from build123d import *
from build123d.topology import SkipClean

# Parameters (mm, degrees)
SKETCH_1_R          = 7.75
EXTRUDE_1_DEPTH     = 1.5
SKETCH_2_R          = 6.5
EXTRUDE_2_DEPTH     = 4
SKETCH_4_W          = 19
SKETCH_4_H          = 19
CUT_EXTRUDE_1_DEPTH = 1
SKETCH_5_R          = 0.4
EXTRUDE_3_DEPTH     = 5.1
FILLET_1_R          = 0.4
FILLET_2_R          = 1


with BuildPart() as part:
    # 草图1 → 凸台-拉伸1 (new body)
    with BuildSketch(Plane.XY):
        Circle(SKETCH_1_R)
    extrude(amount=EXTRUDE_1_DEPTH)

    # 草图2 → 凸台-拉伸2 (add)
    with BuildSketch(Plane.XY.offset(1.5)):
        Circle(SKETCH_2_R)
    extrude(amount=EXTRUDE_2_DEPTH)

    # 草图4 → 切除-拉伸1 (cut)
    with BuildSketch(Plane.XY.offset(5.5)):
        Rectangle(SKETCH_4_W, SKETCH_4_H)
        Polygon((-2.5, 7.5), (-2.5, 2.5), (-7.5, 2.5), (-7.5, -2.5), (-2.5, -2.5), (-2.5, -7.5), (2.5, -7.5), (2.5, -2.5), (7.5, -2.5), (7.5, 2.5), (2.5, 2.5), (2.5, 7.5), align=None, mode=Mode.SUBTRACT)
    extrude(amount=-CUT_EXTRUDE_1_DEPTH, mode=Mode.SUBTRACT)

    # 草图3 → 切除-旋转2 (revolve, cut)
    with SkipClean():  # the faces are left unmerged after this step: merging them gives an invalid solid
        with BuildSketch(Plane(origin=(0, 0, 0), x_dir=(1, 0, 0), z_dir=(0, 1, 0)), mode=Mode.PRIVATE) as cut_revolve_2_sk:
            with BuildLine():
                Line((-6.5, -5.5), (0, -5.5))
                Line((0, -5.5), (0, -4.735087663))
                ThreePointArc((0, -4.735087663), (-3.272426122, -4.926973248), (-6.5, -5.5))
            make_face()
            with BuildLine():
                Line((0, -4.735087663), (0, -5.5))
                Line((0, -5.5), (6.5, -5.5))
                ThreePointArc((6.5, -5.5), (3.272426122, -4.926973248), (0, -4.735087663))
            make_face()
        revolve(cut_revolve_2_sk.sketch.rotate(Axis((0, 0, 1000), (0, 0, -1)), 337.380135052), axis=Axis((0, 0, 1000), (0, 0, -1)), mode=Mode.SUBTRACT)
    add(part.part.scale(1), mode=Mode.REPLACE)  # the faces are merged on a copy

    # 草图5 → 凸台-拉伸3 (add)
    with BuildSketch(Plane(origin=(0, 0, 0), x_dir=(-1, 0, 0), z_dir=(0, 0, -1))):
        Circle(SKETCH_5_R)
    extrude(amount=-EXTRUDE_3_DEPTH)

    # 圆角1
    # the kernel refuses this fillet: 0.4 mm, written as the material it takes off along each edge
    with BuildSketch(Plane(origin=(0, 0, 5.1), x_dir=(-1, 0, 0), z_dir=(0, -1, 0))) as fillet_1_piece_1:
        with BuildLine():
            CenterArc((0.001803842, 0.4), FILLET_1_R, 270, 84.556601085)
            Line((0.001803842, 0), (0.001803842, -0.008))
            Line((0.001803842, -0.008), (0.4, -0.008))
            Line((0.4, -0.008), (0.408, 0))
            ThreePointArc((0.408, 0), (0.408, 0.181027524), (0.407963923, 0.36129615))
            Line((0.407963923, 0.36129615), (0.4, 0.362055049))
        make_face()
    revolve(axis=Axis((0, 0, 5.1), (0, 0, -1)), mode=Mode.SUBTRACT)

    # 圆角2
    fillet_2_edges = [part.edges().sort_by_distance(p)[0] for p in [
        (2.5, 2.5, 4.729599419),
        (2.5, -2.5, 4.729599419),
        (-2.5, -2.5, 4.729599419),
        (-2.5, 2.5, 4.729599419),
    ]]
    fillet(fillet_2_edges, radius=FILLET_2_R)


solid = part.part
For this review, take the finished solid that the model builds, in its own axes (mm). A direction names the side the tool comes from. Give positions to 0.01 mm unless a question says otherwise; leave off trailing zeros. Order: outer loops, then holes, each group sorted by start corner. A loop starts at its lowest first (then second) coordinate and runs counter-clockwise, first axis right, second up. Notation, with made-up numbers: M 48.5,17 L 102.5,17 A23 ccw 102.5,46 Z; hole C 43.25,-15 d11. An arc over 180 degrees is marked long. Answer in a Markdown table with one row per item. Add a question column.
(1) Mouldability with a two-part tool opening along Z and no side actions: class faces 6 (the face through (0, 0, 0)), 7 (the face through (4, 4, 4.5)), 8 (the face through (-5, -2.5, 5)) as +Z half, -Z half, draft (parallel to the pull), parting line (faces both ways), or undercut.
(2) Consider section C-C on z = 3.4. State the section outline as (x, y) points.
(3) Consider section D-D on y = -5. State the section outline as (x, z) points.
(4) For faces 1 (the face through (5, -2.5, 5)), 2 (the face through (6.2, 1.95, 3.47)), 3 (the face through (-2.801, 2.785, 4.78)), 4 (the face through (-2.785, -2.801, 4.78)), 5 (the face through (5, 2.5, 5)), list the 3-axis set-ups (+Z, -Z, +X, -X, +Y, -Y) from which the entire face can be reached by the end or side of a thin tool; tool diameter is ignored.
(5) Consider section A-A on y = 4.25. State the section outline as (x, z) points, and give its area (3 significant figures).
(6) Consider section B-B on x = 1.75. State the section outline as (y, z) points.
(7) For pin 1 (1 mm diameter, centred on x = -4.5, y = -4.5, fed in from +Z); pin 2 (1 mm diameter, centred on x = 4, y = 4, fed in from -Z); pin 3 (5 mm diameter, centred on x = -2.5, y = 2, fed in from +Z); pin 4 (0.8 mm diameter, centred on x = 4.5, z = 5, fed in from -Y), all flat-tipped, find the tip position at first contact; note any pin that passes through.
(8) Wall thickness on probe 1 along Z at (x, y) = (3.5, 3.5); probe 2 along Z at (x, y) = (6.75, 0.75); probe 3 along Y at (x, z) = (0, 3.2): over which ranges is each line inside the solid? List them lowest first. Write a range as [from, to].
Evaluation:
| question | item | result |
|---|---|---|
| 1 | face 6 | -Z half |
| 1 | face 7 | +Z half |
| 1 | face 8 | draft |
| 2 | outline | C 0,0 d13 |
| 3 | outline | M -5.92,0 L 5.92,0 L 5.92,1.5 L 4.15,1.5 L 4.15,4.5 L 2.5,4.5 L 2.5,5.3 A27.55 cw -2.5,5.3 L -2.5,4.5 L -4.15,4.5 L -4.15,1.5 L -5.92,1.5 Z |
| 4 | face 1 | +Z, +X, -Y |
| 4 | face 2 | +Z |
| 4 | face 3 | +Z, -X, +Y |
| 4 | face 4 | +Z, -X, -Y |
| 4 | face 5 | +Z, +X, +Y |
| 5 | outline | M -6.48,0 L 6.48,0 L 6.48,1.5 L 4.92,1.5 L 4.92,4.5 L 2.5,4.5 L 2.5,5.17 A27.68 cw -2.5,5.17 L -2.5,4.5 L -4.92,4.5 L -4.92,1.5 L -6.48,1.5 Z |
| 5 | area | 51.9 mm^2 |
| 6 | outline | M -7.55,0 L 7.55,0 L 7.55,1.5 L 6.26,1.5 L 6.26,5.5 A27.95 cw -6.26,5.5 L -6.26,1.5 L -7.55,1.5 Z |
| 7 | pin 1 | stops at z = 4.5 |
| 7 | pin 2 | stops at z = 0 |
| 7 | pin 3 | stops at z = 5.29 |
| 7 | pin 4 | stops at y = -2.5 |
| 8 | probe 1 | z = [0, 4.5] |
| 8 | probe 2 | z = [0, 1.5] |
| 8 | probe 3 | y = [-6.5, 6.5] |
